Design review of the part built by this model. Coordinates are the model's own, in mm. Coordinates: 2 decimals unless noted, no trailing zeros. Loops run counter-clockwise (first coordinate to the right, second up) from the corner with the lowest first, then second, coordinate; pieces in that order, holes last. Notation, with made-up numbers: M 24.5,12 L 48.5,12 A26 cw 48.5,37 Z; hole C 14,63.25 d7. An arc over 180 degrees is marked long. Write item = value, one per line. Start each with the question number.
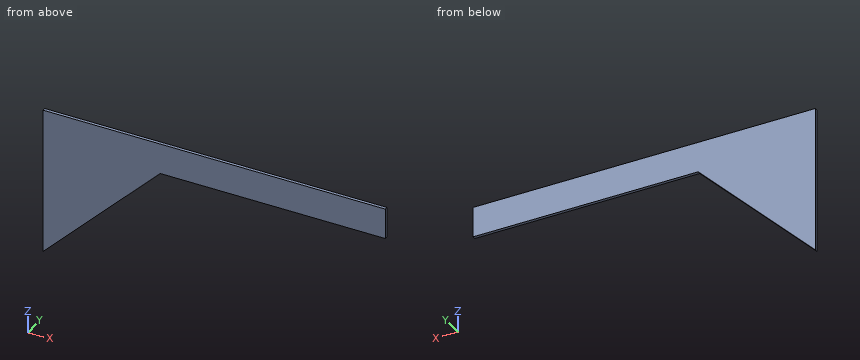
from build123d import *

# Parameters (mm, degrees)
BOSS_EXTRUDE1_DEPTH = 3.175


with BuildPart() as part:
    # Sketch1 → Boss-Extrude1 (new body)
    with BuildSketch(Plane(origin=(0, 0, 0), x_dir=(1, 0, 0), z_dir=(0, 1, 0))):
        Polygon((152.4, 0), (0, 0), (0, 152.4), align=None)
        Polygon((120.65, 31.75), (152.4, 0), (352.425, 0), (352.425, 31.75), align=None)
    extrude(amount=BOSS_EXTRUDE1_DEPTH)


solid = part.part
Q1. Add section C-C on z = -136. State the section outline as (x, y) points (3 decimals).
Q2. Add section B-B on x = 34.5. State the section outline as (y, z) points (3 decimals).
Q3. Add section A-A on y = 1.65. State the section outline as (x, z) points (3 decimals), plus the area to 3 significant figures.
Q4. To check wall thickness, follow line 1 (Z direction, x = 267, y = 1.45); line 2 (Z direction, x = 36.5, y = 2.5); line 3 (X direction, y = 1.5, z = -119.5). State the ranges of each line that lie inside material, in increasing order. Write a range as from..to.
Values follow:
q1.outline = M 0,0 L 16.4,0 L 16.4,3.175 L 0,3.175 Z
q2.outline = M 0,-117.9 L 3.175,-117.9 L 3.175,0 L 0,0 Z
q3.outline = M 0,-152.4 L 120.65,-31.75 L 352.425,-31.75 L 352.425,0 L 0,0 Z
q3.area = 18,500 mm2
q4.line_1 = -31.75..0
q4.line_2 = -115.9..0
q4.line_3 = 0..32.9
